Check sheet for the drawn part. Datum: minimum x, y, z corner. Units: mm. A direction names the side the tool comes from. Round coordinates to 2 decimals unless told otherwise and drop trailing zeros. Write each loop counter-clockwise with the first axis right and the second up, starting at its lowest first coordinate (ties: lowest second). Pieces come first, ordered by that corner, then holes. Notation, with made-up numbers: M 1,6 L 60,6 A24 cw 60,25 Z; hole C -35,15.25 d7. An arc over 180 degrees is marked long. One line per item, written item: value. Start each with the question number.
Item 1: Thickness scan on probe 1 along Z at (x, y) = (6.5, 4.25) (1 decimal); probe 2 along X at (y, z) = (5.2, 9.75) (1 decimal); probe 3 along X at (y, z) = (4.8, 2) (1 decimal). Record the ranges inside material, lowest first. Write a range as from..to.
Item 2: Gauge pin test, flat end, axial feed: pin 1 (2.5 mm diameter, centred on x = 8, z = 7, fed in from -Y). Record the tip position at first contact, or that the pin passes through.
Item 3: Section check C-C, the plane z = 6.5. Record the cut outline in (x, y) (1 decimal).
Item 4: Section check A-A, the plane y = 4.4. State how many separate pieces and enclosed holes the cut face has, then the cut area to 3 significant figures.
Item 5: Draft check along Z on the marked faces 3, 4 and 5. Enter one of: +Z half, -Z half, draft (parallel to the pull), parting line (faces both ways), or undercut.
Item 6: Section check B-B, the plane x = 6.75. Record the cut outline in (y, z) (1 decimal), then the cut area to 3 significant figures.
Item 7: Tool access check on the marked faces 1 and 2. Record the directions out of +Z, -Z, +X, -X, +Y, -Y that give a thin tool (end or side, any length) a straight path to the whole face; none if there is none.
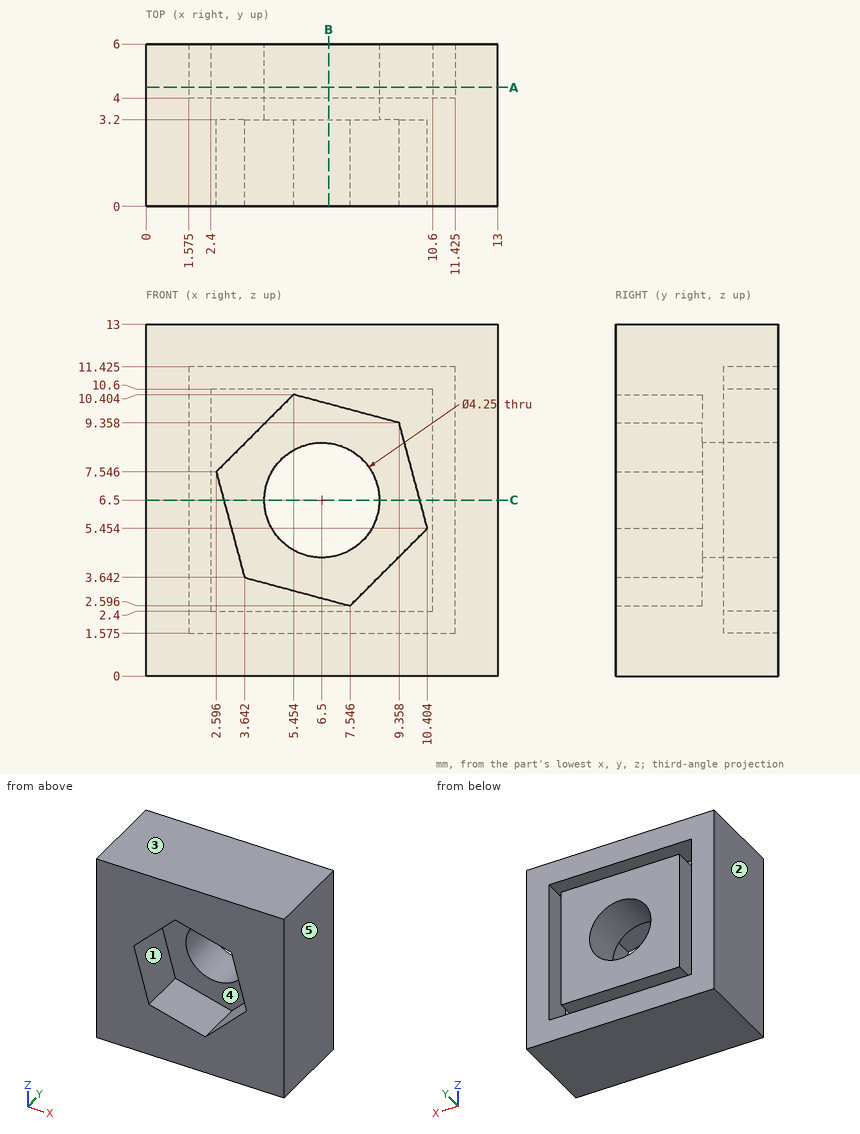
Response values:
1. probe 1: z = 0..1.6, 2.4..4.4, 8.6..10.6, 11.4..13
1. probe 2: x = 0..1.6, 2.4..10.6, 11.4..13
1. probe 3: x = 0..1.6, 11.4..13
2. pin 1: stops at y = 3.2
3. outline: M 0,0 L 2.9,0 L 2.9,3.2 L 4.4,3.2 L 4.4,6 L 2.4,6 L 2.4,4 L 1.6,4 L 1.6,6 L 0,6 Z; M 8.6,3.2 L 10.1,3.2 L 10.1,0 L 13,0 L 13,6 L 11.4,6 L 11.4,4 L 10.6,4 L 10.6,6 L 8.6,6 Z
4. separate pieces: 2
4. enclosed holes: 2
4. area: 125 mm2
5. face 3: +Z half
5. face 4: undercut
5. face 5: draft
6. outline: M 0,0 L 6,0 L 6,1.6 L 4,1.6 L 4,2.4 L 6,2.4 L 6,4.4 L 3.2,4.4 L 3.2,2.8 L 0,2.8 Z; M 0,10.1 L 3.2,10.1 L 3.2,8.6 L 6,8.6 L 6,10.6 L 4,10.6 L 4,11.4 L 6,11.4 L 6,13 L 0,13 Z
6. area: 39.7 mm2
7. face 1: -Y
7. face 2: +Z, -Z, -X, +Y, -Y
